Can you work these out from the model? Positions are in its coordinate system, mm. A direction names the side the tool comes from. Give positions to 0.01 mm unless a question says otherwise; leave off trailing zeros. Order: outer loops, then holes, each group sorted by start corner. A loop starts at its lowest first (then second) coordinate and runs counter-clockwise, first axis right, second up. Notation, with made-up numbers: M -3.75,45.25 L 48.25,45.25 A19 cw 48.25,57.25 Z; hole C -25,-20 d11. An arc over 180 degrees is marked long. Use one line per item in the form item = value. Start each with the question number.
1. I want a section at A-A, the plane y = 18. List the corners of the cut face in (x, z) for me.
2. I want a section at B-B, the plane y = -26. List the corners of the cut face in (x, z) for me, and give its area (3 significant figures).
3. I want a section at C-C, the plane x = 30.5. List the corners of the cut face in (y, z) for me.
4. We'd pull the mould along Y, two halves only. Please class faces 1 (the face through (-1, 0, -5)), 2 (the face through (42, -38, 0)), 3 (the face through (-49.997, 6.631, 0.07)), 4 (the face through (49, 46, 0)): +Y half, -Y half, draft (parallel to the pull), parting line (faces both ways), or undercut.
5. I need wall thicknesses on L1, parallel to Y at x = 52, z = -2; L2, parallel to Z at x = -18, y = -41; L3, parallel to X at y = -24.5, z = 2. Which ranges of each line are inside material? Lowest first, please.
6. Will these pins go through, and if not, where does the flat tip stop? P1, Ø4, axis at x = 35.5, z = -0.5, coming from the +Y side; P2, Ø5, axis at x = -42, z = 0, coming from the +Y side; P3, Ø3, axis at x = -17.5, y = 35, coming from the +Z side.
7. I want a section at D-D, the plane y = 62. List the corners of the cut face in (x, z) for me, and give its area (3 significant figures).
8. For faces 5 (the face through (-15.83, 35.64, -0.89)), 6 (the face through (-19.6, -42.1, -1.2)), 7 (the face through (36, 58, 0)), 8 (the face through (-49, 46, 0)), which set-ups out of +Z, -Z, +X, -X, +Y, -Y let a thin tool reach every point of the face, with its end or its side?
Autodesk Inventor part; units mm, degrees
ref_plane "YZ Plane" through (0, 0, 0) normal (1, 0, 0) x (0, 1, 0)
ref_plane "XZ Plane" through (0, 0, 0) normal (0, 1, 0) x (-1, 0, 0)
ref_plane "XY Plane" through (0, 0, 0) normal (0, 0, 1) x (1, 0, 0)
sketch "Sketch1" plane through (0, 0, 0) normal (0, 0, 1) x (1, 0, 0)
  line L0 (-60, -46) -> (60, -46)
  line L1 (60, -46) -> (60, 46)
  line L2 (60, 46) -> (-60, 46)
  line L3 (-60, 46) -> (-60, -46)
  line L4 (-60, -46) -> (60, 46) construction
  line L5 (60, -46) -> (-60, 46) construction
  point P0 (0, 0)
  dimension "d0" = 120
  dimension "d1" = 92
extrude "Extrusion1" add sketch "Sketch1" along normal mid plane 10
sketch "Sketch2" plane through (0, 0, 5) normal (0, 0, 1) x (1, 0, 0)
  circle A0 centre (0, 18) radius 7
  line L0 (-60, -46) -> (60, -46)
  circle A1 centre (-10.6066, 28.6066) radius 2.1
  circle A2 centre (-15.5563, 33.5563) radius 2.1
  circle A3 centre (-15.5563, 2.4437) radius 2.1
  circle A4 centre (-10.6066, 7.3934) radius 2.1
  circle A5 centre (15.5563, 2.4437) radius 2.1
  circle A6 centre (10.6066, 7.3934) radius 2.1
  circle A7 centre (15.5563, 33.5563) radius 2.1
  circle A8 centre (10.6066, 28.6066) radius 2.1
  line L1 (-15.5563, 33.5563) -> (0, 18) construction
  line L2 (0, 18) -> (-10.6066, 18) construction
  point P0 (0, 0)
  point P1 (0, -46)
  dimension "d4" = 14
  dimension "d6" = 64
  dimension "d7" = 4.2
  dimension "d9" = 15
  dimension "d10" = 4.2
  dimension "d14" = 360
  dimension "d118" = 45
  dimension "d119" = 22
extrude "Extrusion2" cut sketch "Sketch2" against normal through all contours A0 | A2 | A3 | A5 | A7
sketch "Sketch5" plane through (0, 0, 5) normal (0, 0, 1) x (1, 0, 0)
  line L0 (-60, -46) -> (60, -46)
  line L1 (-8.6188, -46) -> (-4, -38)
  line L2 (-4, -38) -> (4, -38)
  line L3 (4, -38) -> (8.6188, -46)
  point P0 (0, 0)
  point P1 (0, -38)
  point P2 (0, -46)
  dimension "d42" = 8
  dimension "d43" = 8
  dimension "d44" = 60
extrude "Extrusion5" cut sketch "Sketch5" against normal through all
sketch "Sketch7" plane through (60, -46, -5) normal (0, -1, 0) x (1, 0, 0)
  circle A0 centre (-6, 5) radius 2
  line L0 (0, 0) -> (-51.3812, 0) construction
  circle A1 centre (-18, 5) radius 2
  circle A2 centre (-30, 5) radius 2
  circle A3 centre (-42, 5) radius 2
  circle A4 centre (-54, 5) radius 2 construction
  circle A5 centre (-66, 5) radius 2 construction
  circle A6 centre (-78, 5) radius 2
  circle A7 centre (-90, 5) radius 2
  circle A8 centre (-102, 5) radius 2
  circle A9 centre (-114, 5) radius 2
  line L1 (-54, 5) -> (-66, 5) construction
  point P0 (-60, 5)
  point P1 (-60, 5)
  dimension "d74" = 4
  dimension "d77" = 12
extrude "Extrusion7" cut sketch "Sketch7" against normal blind 8
sketch "Sketch8" plane through (0, 0, 5) normal (0, 0, 1) x (1, 0, 0)
  circle A0 centre (-52, 38) radius 2.1
  line L0 (-60, 46) -> (-60, -46) construction
  line L1 (-60, -46) -> (-8.6188, -46)
  circle A1 centre (-52, 6) radius 2.1
  circle A2 centre (-52, -26) radius 2.1
  circle A3 centre (0, 18) radius 7 construction
  line L2 (0, 25) -> (0, 18) construction
  circle A4 centre (52, 38) radius 2.1
  circle A5 centre (52, 6) radius 2.1
  circle A6 centre (52, -26) radius 2.1
  point P0 (0, 0)
  dimension "d84" = 4.2
  dimension "d85" = 8
  dimension "d86" = 84
  dimension "d89" = 32
extrude "Extrusion8" cut sketch "Sketch8" against normal through all
sketch "Sketch9" plane through (0, 0, 5) normal (0, 0, 1) x (1, 0, 0)
  line L0 (-36, 46) -> (36, 46)
  line L1 (36, 46) -> (36, 70)
  line L2 (36, 70) -> (-36, 70)
  line L3 (-36, 70) -> (-36, 46)
  line L4 (-36, 46) -> (36, 70) construction
  line L5 (36, 46) -> (-36, 70) construction
  line L6 (60, 46) -> (-60, 46) construction
  point P0 (0, 0)
  point P1 (0, 58)
  point P2 (0, 46)
  dimension "d96" = 72
  dimension "d97" = 24
extrude "Extrusion9" add sketch "Sketch9" against normal up to surface (10 mm away)
sketch "Sketch10" plane through (0, 0, 5) normal (0, 0, 1) x (1, 0, 0)
  circle A0 centre (0, 18) radius 7 construction
  circle A1 centre (-17, 62) radius 2.1
  line L0 (-7, 18) -> (0, 18) construction
  line L1 (0, 18) -> (0, 25) construction
  circle A2 centre (17, 62) radius 2.1
  circle A3 centre (-17, -26) radius 2.1
  circle A4 centre (17, -26) radius 2.1
  point P0 (0, 0)
  dimension "d100" = 4.2
  dimension "d101" = 44
  dimension "d102" = 17
extrude "Extrusion10" cut sketch "Sketch10" against normal blind 10
fillet "Fillet1" radius 10 4 edges at (36, 46, 0) (-36, 46, 0) (-36, 70, 0) (36, 70, 0)
fillet "Fillet2" radius 8 2 edges at (-60, 46, 0) (60, 46, 0)
thread "Thread9"
thread "Thread10"
hole "Hole1" at (-15.5563, 33.5563, 5) at (-15.5563, 2.4437, 5) at (15.5563, 2.4437, 5) at (15.5563, 33.5563, 5) direction (0, 0, -1) diameter 4.2 end through all countersink diameter 8 countersink angle 90
properties part number "FirstStageMotorMountingPlate" material "Aluminum 6061"
Check result:
q1.outline = M -60,-5 L -7,-5 L -7,5 L -60,5 Z; M 7,-5 L 60,-5 L 60,5 L 7,5 Z
q2.outline = M -60,-5 L -54.1,-5 L -54.1,5 L -60,5 Z; M -49.9,-5 L -19.1,-5 L -19.1,5 L -49.9,5 Z; M -14.9,-5 L 14.9,-5 L 14.9,5 L -14.9,5 Z; M 19.1,-5 L 49.9,-5 L 49.9,5 L 19.1,5 Z; M 54.1,-5 L 60,-5 L 60,5 L 54.1,5 Z
q2.area = 1,030 mm2
q3.outline = M -46,-5 L 68.93,-5 L 68.93,5 L -46,5 L -46,1.94 L -38,1.94 L -38,-1.94 L -46,-1.94 Z
q4.face_1 = draft
q4.face_2 = -Y half
q4.face_3 = undercut
q4.face_4 = +Y half
q5.L1 = -46 to -28.1, -23.9 to 3.9, 8.1 to 35.9, 40.1 to 46
q5.L2 = -5 to -2, 2 to 5
q5.L3 = -60 to -53.47, -50.53 to -18.47, -15.53 to 15.53, 18.47 to 50.53, 53.47 to 60
q6.P1 = 66.61
q6.P2 = 48.4
q6.P3 = 4.92
q7.outline = M -35.8,-5 L -19.1,-5 L -19.1,5 L -35.8,5 Z; M -14.9,-5 L 14.9,-5 L 14.9,5 L -14.9,5 Z; M 19.1,-5 L 35.8,-5 L 35.8,5 L 19.1,5 Z
q7.area = 632 mm2
q8.face_5 = +Z, -Z
q8.face_6 = -Y
q8.face_7 = +Z, -Z, +X, +Y
q8.face_8 = +Z, -Z, -X, +Y
